Answer from the drawing. Dimensions are ordinates in mm from the lowest x, y and z of the part. A direction names the side the tool comes from. Round coordinates to 2 decimals unless told otherwise and drop trailing zeros. Order: outer loops, then holes, each group sorted by start corner. A loop starts at its lowest first (then second) coordinate and runs counter-clockwise, first axis right, second up.
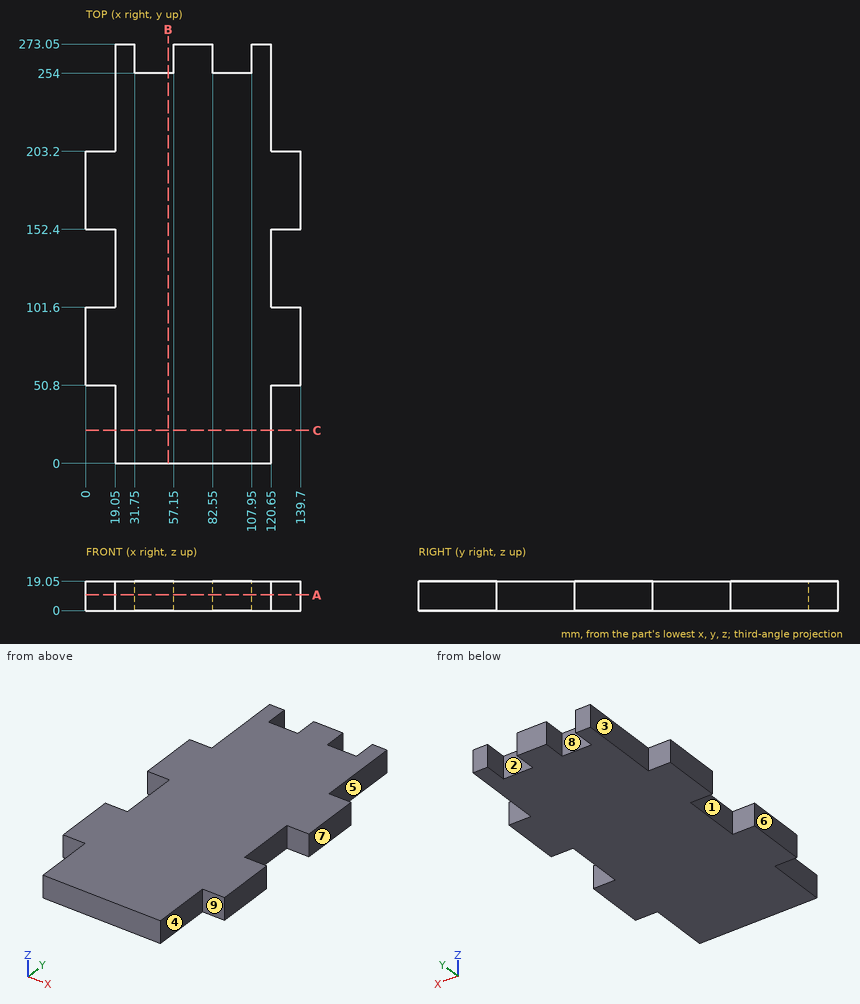
Q1. For the marked faces 1, 2, 3, 4 and 5, determine the directions among +Z, -Z, +X, -X, +Y, -Y from which every point of the face is accessible in a straight line to the end or side of a thin tool.
Outcome:
face 1: +Z, -Z, -X
face 2: +Z, -Z, +Y
face 3: +Z, -Z, -X, +Y
face 4: +Z, -Z, +X, -Y
face 5: +Z, -Z, +X, +Y
Q2. Flat-ended cylindrical pins translate along their axes: pin 1 (10 mm diameter, centred on x = 86.5, y = 151, fed in from -Z); pin 2 (5.5 mm diameter, centred on y = 266.5, z = 7, fed in from +X); pin 3 (9.5 mm diameter, centred on x = 128.5, z = 13.5, fed in from +Y); pin 4 (9.5 mm diameter, centred on x = 10, z = 7, fed in from -Y). Find the tip coordinate at first contact, or state that the pin passes through.
Outcome:
pin 1: stops at z = 0
pin 2: stops at x = 120.65
pin 3: stops at y = 203.2
pin 4: stops at y = 50.8
Q3. A cutting plane is placed at C-C, the plane y = 21.5. Give the vertices of the cut face in (x, z).
Outcome:
outline: (19.05, 0) - (120.65, 0) - (120.65, 19.05) - (19.05, 19.05) - close
Q4. For a pull along X with two mould halves and no side action, classify the marked faces 6, 7, 8 and 9 as released by +X, released by -X, zero draft, split by the parting line, or undercut.
Outcome:
face 6: released by -X
face 7: released by +X
face 8: undercut
face 9: zero draft
Q5. Straight lines are drawn through the part: probe 1 along X at (y, z) = (261, 16); probe 2 along X at (y, z) = (204, 5.5); probe 3 along Y at (x, z) = (54.5, 13.75). For each, find the intervals that lie inside material, in ascending order.
Outcome:
probe 1: x = 19.05 to 31.75, 57.15 to 82.55, 107.95 to 120.65
probe 2: x = 19.05 to 120.65
probe 3: y = 0 to 254
Q6. A cutting plane is placed at A-A, the plane z = 10.25. Give the vertices of the cut face in (x, y).
Outcome:
outline: (0, 50.8) - (19.05, 50.8) - (19.05, 0) - (120.65, 0) - (120.65, 50.8) - (139.7, 50.8) - (139.7, 101.6) - (120.65, 101.6) - (120.65, 152.4) - (139.7, 152.4) - (139.7, 203.2) - (120.65, 203.2) - (120.65, 273.05) - (107.95, 273.05) - (107.95, 254) - (82.55, 254) - (82.55, 273.05) - (57.15, 273.05) - (57.15, 254) - (31.75, 254) - (31.75, 273.05) - (19.05, 273.05) - (19.05, 203.2) - (0, 203.2) - (0, 152.4) - (19.05, 152.4) - (19.05, 101.6) - (0, 101.6) - close
Q7. A cutting plane is placed at B-B, the plane x = 53.5. Give the vertices of the cut face in (y, z).
Outcome:
outline: (0, 0) - (254, 0) - (254, 19.05) - (0, 19.05) - close
